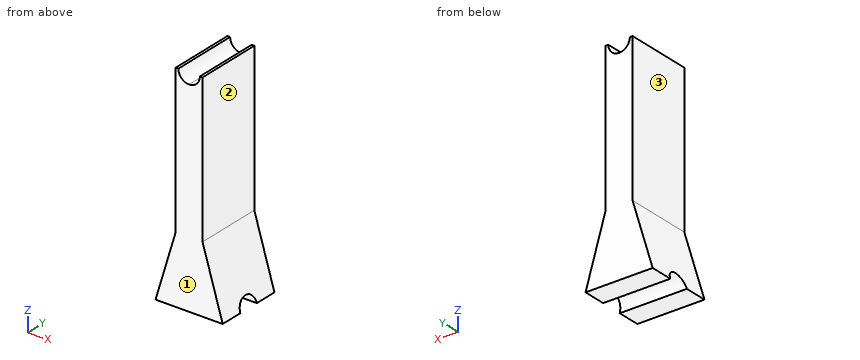
from build123d import *

# Parameters (mm, degrees)
F1_DEPTH = 25
F4_DEPTH = 30
F5_DEPTH = 15


with BuildPart() as f1:
    # F0 (on Front) → F1 (new body)
    with BuildSketch(Plane.XZ):
        Polygon((0, 80), (0, 0), (12.5, 0), (5, 25), (5, 80), align=None)
    extrude(amount=F1_DEPTH)

    # F3 (on face) → F4 (cut)
    with BuildSketch(Plane.XZ.offset(25)):
        with BuildLine():
            ThreePointArc((0, 76), (2.828427, 77.171573), (4, 80))
            Line((4, 80), (0, 80))
            Line((0, 80), (0, 76))
        make_face()
    extrude(amount=-F4_DEPTH, mode=Mode.SUBTRACT)

    # F2 (on face) → F5 (cut)
    with BuildSketch(Plane(origin=(0, 0, 0), x_dir=(0, -1, 0), z_dir=(-1, 0, 0))):
        with BuildLine():
            Line((8.5, 0), (16.5, 0))
            ThreePointArc((16.5, 0), (12.5, 4), (8.5, 0))
        make_face()
    extrude(amount=-F5_DEPTH, mode=Mode.SUBTRACT)

    # F6: F1 across plane


with BuildPart() as f1_1:
    add(f1.part)
    add(f1.part.mirror(Plane.YZ))


solid = f1_1.part
Verification items for the finished model (mm, model axes). Face numbers are marked on the shaded views. A direction names the side the tool comes from. Give positions to 0.01 mm unless a question says otherwise; leave off trailing zeros. Loops run counter-clockwise (first coordinate to the right, second up) from the corner with the lowest first, then second, coordinate; pieces in that order, holes last.
1. Material ranges on probe 1 along X at (y, z) = (-21.25, 53); probe 2 along X at (y, z) = (-19, 9); probe 3 along Z at (x, y) = (-0.5, -11.75), recorded low to high.
Derived:
probe 1: x = -5 to 5
probe 2: x = -9.8 to 9.8
probe 3: z = 3.93 to 76.03
2. Tool access check on the marked faces 1, 2 and 3. Record the directions out of +Z, -Z, +X, -X, +Y, -Y that give a thin tool (end or side, any length) a straight path to the whole face; none if there is none.
Derived:
face 1: +Z, -Z, +X, -X, -Y
face 2: +Z, +X, +Y, -Y
face 3: +Z, -X, +Y, -Y
3. Go/stop test with flat-tipped pins: P1, Ø5, axis at y = -7.5, z = 50.5, coming from the -X side; P2, Ø12, axis at y = -2.5, z = 48, coming from the +X side; P3, Ø10, axis at y = -7, z = 26.5, coming from the -X side. Record where each tip stops, or that it passes through.
Derived:
P1: stops at x = -5
P2: stops at x = 5
P3: stops at x = -6.05
4. Cross-section at C-C on y = -12.5. Record the cut outline in (x, z).
Derived:
outline: (-11.3, 4) - (11.3, 4) - (5, 25) - (5, 80) - (4, 80) arc R4 cw to (-4, 80) - (-5, 80) - (-5, 25) - close
5. Cross-section at B-B on x = -10.25. Record the cut outline in (y, z), and give its area (3 significant figures).
Derived:
outline: (-25, 0) - (-16.5, 0) arc R4 cw to (-8.5, 0) - (0, 0) - (0, 7.5) - (-25, 7.5) - close
area: 162 mm2
6. Cross-section at A-A on y = -22. Record the cut outline in (x, z), and give its area (3 significant figures).
Derived:
outline: (-12.5, 0) - (12.5, 0) - (5, 25) - (5, 80) - (4, 80) arc R4 cw to (-4, 80) - (-5, 80) - (-5, 25) - close
area: 962 mm2
7. Cross-section at D-D on z = 57. Record the cut outline in (x, y), and give its area (3 significant figures).
Derived:
outline: (-5, -25) - (5, -25) - (5, 0) - (-5, 0) - close
area: 250 mm2
